Job drawing, mm, ordinate dimensions from the low corner. One solid piece. A direction names the side the tool comes from. Give positions to 0.01 mm unless a question says otherwise; leave off trailing zeros. Write each loop counter-clockwise with the first axis right and the second up, starting at its lowest first coordinate (ties: lowest second). Pieces come first, ordered by that corner, then holes. Notation, with made-up numbers: M 61.25,10 L 73.25,10 A21 ccw 73.25,22 Z; hole C -1.5,-24 d9. An arc over 180 degrees is marked long. Use a Markdown table: item, result.
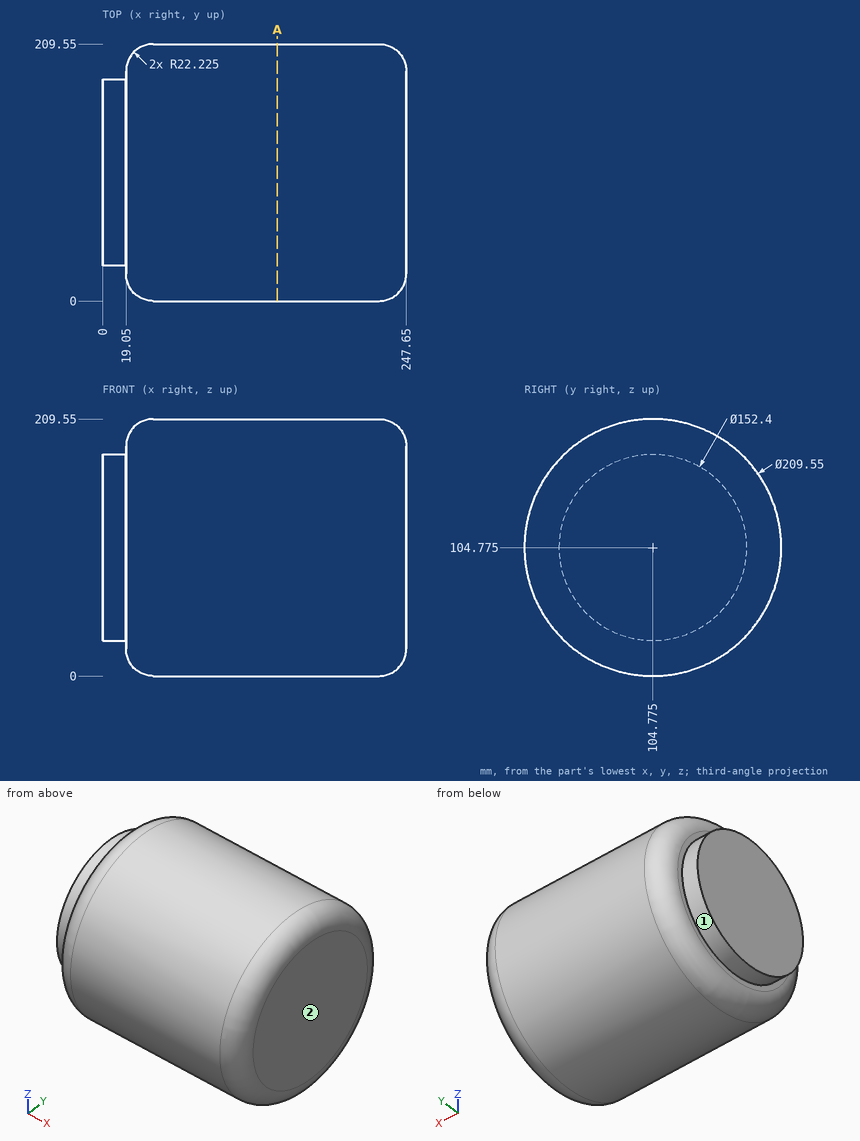
1. Drop flat-ended pins along their axis: P1, Ø1, axis at x = 32.5, y = 88.5, coming from the +Z side; P2, Ø8, axis at x = 47, z = 115, coming from the -Y side; P3, Ø8, axis at x = 54.5, z = 144, coming from the +Y side. Give the stop position or say it passes through.
Findings below:
| item | result |
|---|---|
| P1 | z = 206.68 |
| P2 | y = 0.19 |
| P3 | y = 203.45 |
2. Drill centre lines: L1, parallel to X at y = 156.5, z = 48; L2, parallel to X at y = 180, z = 69; L3, parallel to Y at x = 165.5, z = 103. Where is each one in solid material? Low to high.
Findings below:
| item | result |
|---|---|
| L1 | 19.05 to 247.65 |
| L2 | 19.06 to 247.64 |
| L3 | 0.02 to 209.53 |
3. Cut at A-A, the plane x = 142.5. Give the cut face in (y, z) (3 decimals), then the cut area to 3 significant figures.
Findings below:
| item | result |
|---|---|
| outline | C 104.775,104.775 d209.55 |
| area | 34,500 mm2 |
4. Tool access for the marked faces 1 and 2: list every direction of +Z, -Z, +X, -X, +Y, -Y with a clear straight run to the whole face (end or side of a thin tool).
Findings below:
| item | result |
|---|---|
| face 1 | -X |
| face 2 | +Z, -Z, +X, +Y, -Y |
